from build123d import *

# Parameters (mm, degrees)
SKETCH1_W           = 200
SKETCH1_H           = 180
BOSS_EXTRUDE1_DEPTH = 3
SKETCH2_W           = 200
SKETCH2_H           = 140
BOSS_EXTRUDE2_DEPTH = 5
SKETCH6_W           = 200
SKETCH6_H           = 179.869705491
BOSS_EXTRUDE3_DEPTH = 20
SKETCH7_W           = 155
SKETCH7_H           = 20
CUT_EXTRUDE1_DEPTH  = 179.869705491
SKETCH8_R           = 2
BOSS_EXTRUDE4_DEPTH = 155


with BuildPart() as part:
    # Sketch1 → Boss-Extrude1 (new body)
    with BuildSketch(Plane(origin=(0, 0, 0), x_dir=(1, 0, 0), z_dir=(0, 1, 0))):
        Rectangle(SKETCH1_W, SKETCH1_H)
    extrude(amount=BOSS_EXTRUDE1_DEPTH)

    # Sketch2 → Boss-Extrude2 (add)
    with BuildSketch(Plane.XZ):
        with Locations((0, 20)):
            Rectangle(SKETCH2_W, SKETCH2_H)
    extrude(amount=BOSS_EXTRUDE2_DEPTH)

    # Sketch6 → Boss-Extrude3 (add)
    with BuildSketch(Plane(origin=(0, 3, 0), x_dir=(1, 0, 0), z_dir=(0, 1, 0))):
        with Locations((0, -0.065147254)):
            Rectangle(SKETCH6_W, SKETCH6_H)
    extrude(amount=BOSS_EXTRUDE3_DEPTH)

    # Sketch7 → Cut-Extrude1 (cut)
    with BuildSketch(Plane(origin=(0, 0, -89.869705491), x_dir=(-1, 0, 0), z_dir=(0, 0, -1))):
        with Locations((-17.5, 13)):
            Rectangle(SKETCH7_W, SKETCH7_H)
    extrude(amount=-CUT_EXTRUDE1_DEPTH, mode=Mode.SUBTRACT)

    # Sketch8 → Boss-Extrude4 (add)
    with BuildSketch(Plane.ZY.offset(-95)):
        with Locations(Location((-79.869705491, 8.5, 0), (0, 0, 180))):
            Circle(SKETCH8_R)
    extrude(amount=BOSS_EXTRUDE4_DEPTH)


solid = part.part
Geometry: final body of the model. Coordinates: model frame, mm. A direction names the side the tool comes from. Give positions to 0.01 mm unless a question says otherwise; leave off trailing zeros. Write each loop counter-clockwise with the first axis right and the second up, starting at its lowest first coordinate (ties: lowest second). Pieces come first, ordered by that corner, then holes. Notation, with made-up numbers: M -14,59.25 L 15,59.25 A31 ccw 15,89.25 Z; hole C 59.5,43.25 d7. An arc over 180 degrees is marked long. Answer in a Markdown table with one row per item. Add a question column.
(1) Section C-C on y = -2.75. Return loops of the section in (x, z).
(2) Section A-A on x = 37.5. Return loops of the section in (y, z), and give its area (3 significant figures).
(3) Mould query, pull axis X, two halves, no side actions, for faces 3 (the flat face through (100, 9, 1)), 4 (the flat face through (-60, 13, -1)), 5 (the flat face through (-80, 23, -1)). Classes: +X half, -X half, draft (parallel to the pull), parting line (faces both ways), or undercut.
(4) Reachability of faces 1 (the flat face through (-1, -5, 21)), 2 (the flat face through (-1, -2, -50)) from +Z, -Z, +X, -X, +Y, -Y: full face, straight path, thin tool, end or side. Return the list, or none.
(5) Section B-B on y = 18.25. Return loops of the section in (x, z), and give its area (3 significant figures).
(6) Ray query, line 1 (X direction, y = 10, z = 24); line 2 (Y direction, x = 83.5, z = -80); line 3 (Z direction, x = -88, y = 7.25). Return the intervals inside material, ascending.
(7) First-contact query: pin 1 (2.5 mm diameter, centred on x = 29.5, y = -3.5, fed in from -Z); pin 2 (1 mm diameter, centred on x = 38.5, z = -36, fed in from +Y); pin 3 (6 mm diameter, centred on x = 78, y = 14.5, fed in from +Z); pin 4 (4 mm diameter, centred on x = 96.5, y = 10.5, fed in from -Z). Flat tips, straight axial feed; report the tip coordinate or a pass-through.
Result set:
| question | item | result |
|---|---|---|
| 1 | outline | M -100,-50 L 100,-50 L 100,90 L -100,90 Z |
| 2 | outline | M -5,-50 L 0,-50 L 0,-90 L 3,-90 L 3,90 L -5,90 Z; C 8.5,-79.87 d4 |
| 2 | area | 1,250 mm^2 |
| 3 | face 3 | +X half |
| 3 | face 4 | undercut |
| 3 | face 5 | draft |
| 4 | face 1 | +Z, -Z, +X, -X, -Y |
| 4 | face 2 | -Z, +X, -X, -Y |
| 5 | outline | M -100,-89.87 L -60,-89.87 L -60,90 L -100,90 Z; M 95,-89.87 L 100,-89.87 L 100,90 L 95,90 Z |
| 5 | area | 8,090 mm^2 |
| 6 | line 1 | x = -100 to -60, 95 to 100 |
| 6 | line 2 | y = 0 to 3, 6.5 to 10.5 |
| 6 | line 3 | z = -89.87 to 90 |
| 7 | pin 1 | stops at z = -50 |
| 7 | pin 2 | stops at y = 3 |
| 7 | pin 3 | passes through |
| 7 | pin 4 | stops at z = -89.87 |
